The model under review builds one solid part; all positions refer to its coordinate system, in mm. Face numbers are marked on the shaded views. A direction names the side the tool comes from. Coordinates: 2 decimals unless noted, no trailing zeros. Order: outer loops, then holes, each group sorted by start corner. A loop starts at its lowest first (then second) coordinate and runs counter-clockwise, first axis right, second up. Notation, with made-up numbers: M 23,74 L 31,74 A22 ccw 31,112 Z; hole C 63,45.5 d6. An arc over 180 degrees is marked long. Answer in a Markdown table with one row per item.
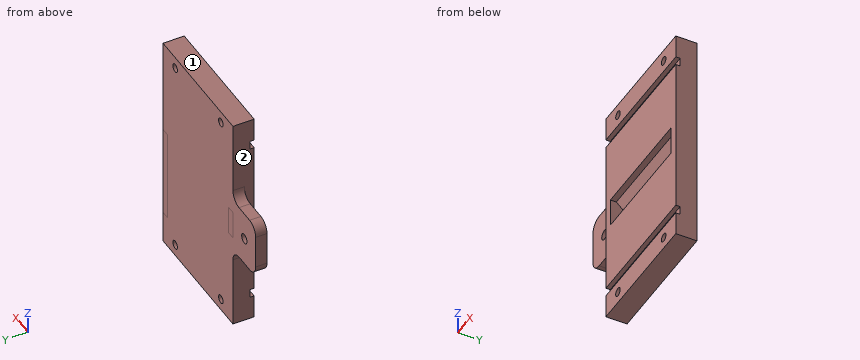
Autodesk Inventor part; units mm, degrees
ref_plane "Work Plane1" through (0, -1.5973, -20.6649) normal (0, 0, 1) x (1, 0, 0)
ref_plane "YZ Plane" through (0, 0, 0) normal (1, 0, 0) x (0, 1, 0)
ref_plane "XZ Plane" through (0, 0, 0) normal (0, 1, 0) x (-1, 0, 0)
sketch "Sketch1" plane through (0, 0, 0) normal (1, 0, 0) x (0, 1, 0)
  line L0 (-1.5973, 19.3351) -> (-9.0973, 19.3351)
  line L1 (-9.0973, -60.6649) -> (-1.5973, -60.6649)
  line L2 (-1.5973, -60.6649) -> (-1.5973, 19.3351)
  line L3 (20.1932, -20.6649) -> (-21.0203, -20.6649)
  line L4 (-9.0973, 19.3351) -> (-9.0973, -15.5649)
  line L5 (-9.0973, -25.7649) -> (-9.0973, -60.6649)
  circle A0 centre (-9.0973, -20.6649) radius 5.1 construction
  line L6 (-11.2098, -15.5649) -> (-6.9848, -15.5649)
  line L7 (-6.9848, -15.5649) -> (-3.9973, -18.5524)
  line L8 (-3.9973, -18.5524) -> (-3.9973, -22.7774)
  line L9 (-3.9973, -22.7774) -> (-6.9848, -25.7649)
  line L10 (-6.9848, -25.7649) -> (-11.2098, -25.7649)
  line L11 (-10.6473, 10.8851) -> (-7.5473, 10.8851)
  line L12 (-7.5473, 10.8851) -> (-7.5473, 7.7851)
  line L13 (-7.5473, 7.7851) -> (-10.6473, 7.7851)
  line L14 (-10.6473, 7.7851) -> (-10.6473, 10.8851)
  line L15 (-10.6473, 10.8851) -> (-7.5473, 7.7851) construction
  line L16 (-7.5473, 10.8851) -> (-10.6473, 7.7851) construction
  point P0 (0, 0)
  point P1 (-9.0973, 9.3351)
  dimension "d6" = 10.2
  dimension "d2" = 7.5
  dimension "d3" = 80
  dimension "d7" = 3.1
  dimension "d9" = 60
extrude "Extrusion1" add sketch "Sketch1" along normal blind 46.2 contours L2 L3 L8 L7 L6 L4 L13 L12 L11 L0 | L2 L1 L5 L10 L9 L8 L3 | L11 L12 L13 L4
extrude "Extrusion2" cut sketch "Sketch1" along normal through all contours L11 L12 L13 L4 | L4 L13 L14 L11
ref_plane "Work Plane1" through (0, -1.5973, -20.6649) normal (0, 0, 1) x (1, 0, 0)
mirror "Mirror1" about plane through (0, -1.5973, -20.6649) normal (0, 0, 1) of "Extrusion2"
sketch "Sketch2" plane through (0, -9.0973, 19.3351) normal (0, -1, 0) x (1, 0, 0)
  line L0 (0, 0) -> (0, -8.45)
  line L1 (0, -4.225) -> (55.9081, -4.225)
  line L2 (0, 0) -> (46.2, 0)
  line L3 (23.1, 0) -> (23.1, -31.5844)
  line L4 (8, 4.0283) -> (8, -8.7646)
  circle A0 centre (8, -4.225) radius 1.5
  circle A1 centre (38.2, -4.225) radius 1.5
  point P0 (0, -19.3351)
  dimension "d12" = 8
  dimension "d13" = 3
extrude "Extrusion3" cut sketch "Sketch2" against normal through all contours A1 L1 | L1 A1 | A0 L4 L1 | L1 L4 A0 | A0 L1 L4 | L1 A0 L4
mirror "Mirror2" about plane through (0, -1.5973, -20.6649) normal (0, 0, 1) of "Extrusion3"
sketch "Sketch3" plane through (0, -9.0973, 19.3351) normal (0, -1, 0) x (1, 0, 0)
  line L0 (0, -68.45) -> (46.2, -68.45)
  line L1 (46.2, -34.9) -> (43.2, -34.9)
  line L2 (43.2, -34.9) -> (43.2, -68.45)
  line L3 (43.2, -68.45) -> (46.2, -68.45)
  line L4 (46.2, -68.45) -> (46.2, -34.9)
  line L5 (0, -34.9) -> (3, -34.9)
  line L6 (3, -34.9) -> (3, -45.1)
  line L7 (3, -45.1) -> (0, -45.1)
  line L8 (0, -45.1) -> (0, -34.9)
  point P0 (0, -19.3351)
  dimension "d16" = 3
  dimension "d17" = 3
extrude "Extrusion4" add sketch "Sketch3" against normal through all
sketch "Sketch4" plane through (0, -1.5973, -60.6649) normal (0, 1, 0) x (1, 0, 0)
  line L0 (0, -50) -> (-15, -50)
  line L1 (-15, -50) -> (-15, -30)
  line L2 (-15, -30) -> (0, -30)
  line L3 (0, -30) -> (0, -50)
  line L4 (58.44, -40) -> (-27.24, -40)
  line L5 (0, 0) -> (0, -80) construction
  circle A0 centre (-7.5, -40) radius 1.75
  point P0 (0, -60.6649)
  dimension "d20" = 15
  dimension "d21" = 20
  dimension "d22" = 3.5
  dimension "d23" = 7.5
extrude "Extrusion5" add sketch "Sketch4" against normal blind 4 contours L0 L1 L4 A0 L3 | L4 A0 L1 L2 L3
fillet "Fillet1" radius 4 4 edges at (0, -3.5973, -10.6649) (-15, -3.5973, -10.6649) (-15, -3.5973, -30.6649) (0, -3.5973, -30.6649)
equation "\"d17\" = d16"
properties part number "PRING_piston_case_half"
(1) Take a section at C-C (x = 24). Write out the cut boundary in (y, z), then the cut area to 3 significant figures.
Report:
| item | result |
|---|---|
| outline | M -9.1,-60.66 L -1.6,-60.66 L -1.6,19.34 L -9.1,19.34 L -9.1,10.89 L -7.55,10.89 L -7.55,7.79 L -9.1,7.79 L -9.1,-15.56 L -6.98,-15.56 L -4,-18.55 L -4,-22.78 L -6.98,-25.76 L -9.1,-25.76 L -9.1,-49.11 L -7.55,-49.11 L -7.55,-52.21 L -9.1,-52.21 Z |
| area | 547 mm^2 |
(2) Insertion check: P1, Ø4, axis at y = -5, z = -10, coming from the -X side; P2, Ø1.5, axis at x = 29, z = 9, coming from the -Y side; P3, Ø3, axis at x = -8.5, y = -4, coming from the -Z side; P4, Ø2.5, axis at x = 38.2, z = -56.44, coming from the +Y side. Each pin has a flat end and moves straight along its axis. Give the tip position at first contact, or say it passes through.
Report:
| item | result |
|---|---|
| P1 | x = -13.98 |
| P2 | y = -7.55 |
| P3 | z = -30.66 |
| P4 | through |
(3) To check wall thickness, follow line 1 (Z direction, x = 15, y = -8); line 2 (Z direction, x = 8, y = -3.25); line 3 (Z direction, x = -7.5, y = -3.1). State the ranges of each line that lie inside material, in increasing order. Write a range as [from, to].
Report:
| item | result |
|---|---|
| line 1 | [-60.66, -52.21], [-49.11, -25.76], [-15.56, 7.79], [10.89, 19.34] |
| line 2 | [-60.66, -57.94], [-54.94, 13.61], [16.61, 19.34] |
| line 3 | [-30.66, -22.41], [-18.91, -10.66] |
(4) Take a section at D-D (z = 0.5). Write out the cut boundary in (x, y).
Report:
| item | result |
|---|---|
| outline | M 0,-9.1 L 46.2,-9.1 L 46.2,-1.6 L 0,-1.6 Z |
(5) Take a section at A-A (x = 8). Write out the cut boundary in (y, z), then the cut area to 3 significant figures.
Report:
| item | result |
|---|---|
| outline | M -9.1,-60.66 L -1.6,-60.66 L -1.6,-57.94 L -9.1,-57.94 Z; M -9.1,-54.94 L -1.6,-54.94 L -1.6,13.61 L -9.1,13.61 L -9.1,10.89 L -7.55,10.89 L -7.55,7.79 L -9.1,7.79 L -9.1,-15.56 L -6.98,-15.56 L -4,-18.55 L -4,-22.78 L -6.98,-25.76 L -9.1,-25.76 L -9.1,-49.11 L -7.55,-49.11 L -7.55,-52.21 L -9.1,-52.21 Z; M -9.1,16.61 L -1.6,16.61 L -1.6,19.34 L -9.1,19.34 Z |
| area | 502 mm^2 |
(6) Take a section at B-B (x = -7.5). Write out the cut boundary in (y, z), then the cut area to 3 significant figures.
Report:
| item | result |
|---|---|
| outline | M -5.6,-30.66 L -1.6,-30.66 L -1.6,-22.41 L -5.6,-22.41 Z; M -5.6,-18.91 L -1.6,-18.91 L -1.6,-10.66 L -5.6,-10.66 Z |
| area | 66.0 mm^2 |
(7) Machinability: for the marked faces 1 and 2, which of the approach directions +Z, -Z, +X, -X, +Y, -Y give a long, thin tool a straight path to every point of the face, cutting with its end or side? Answer none if there is none.
Report:
| item | result |
|---|---|
| face 1 | +Z, +X, -X, +Y, -Y |
| face 2 | -X, -Y |
